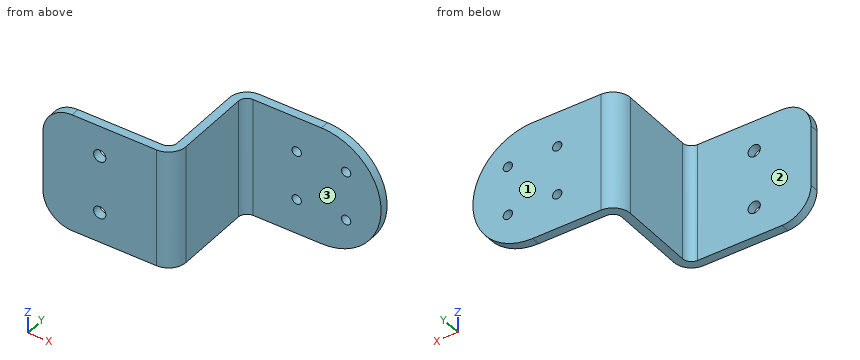
from build123d import *

# Parameters (mm, degrees)
EXTRUDE_THIN1_DEPTH    = 41
CONVERT_SOLID1_DEPTH   = 41
CONVERT_SOLID1_2_DEPTH = 41
SKETCH6_R              = 1.6
CUT_EXTRUDE1_DEPTH     = 3
M5X0_8_TAPPED_HOLE1_D  = 4.2
FILLET1_R              = 10


# Read off the part's stored shape, not the designer's step: Convert-Solid1
with BuildPart() as part:
    # Sketch1 → Extrude-Thin1 (new body)
    with BuildSketch(Plane.XY):
        Polygon((50, 35), (0, 35), (0, 0), (-45, 0), (-45, 3), (-3, 3), (-3, 38), (50, 38), align=None)
    extrude(amount=EXTRUDE_THIN1_DEPTH)

    # Convert-Solid1 outline → Convert-Solid1 (cut)
    with BuildSketch(Plane.XY):
        with BuildLine():
            Line((-3, 38), (-3, 32))
            ThreePointArc((-3, 32), (-1.242640687, 36.242640687), (3, 38))
            Line((3, 38), (-3, 38))
        make_face()
        with BuildLine():
            Line((0, 0), (0, 6))
            ThreePointArc((0, 6), (-1.757359313, 1.757359313), (-6, 0))
            Line((-6, 0), (0, 0))
        make_face()
    extrude(amount=CONVERT_SOLID1_DEPTH, mode=Mode.SUBTRACT)

    # Convert-Solid1 2 outline → Convert-Solid1 2 (add)
    with BuildSketch(Plane.XY):
        with BuildLine():
            Line((-3, 3), (-3, 6))
            ThreePointArc((-3, 6), (-3.878679656, 3.878679656), (-6, 3))
            Line((-6, 3), (-3, 3))
        make_face()
        with BuildLine():
            Line((0, 35), (0, 32))
            ThreePointArc((0, 32), (0.878679656, 34.121320344), (3, 35))
            Line((3, 35), (0, 35))
        make_face()
    extrude(amount=CONVERT_SOLID1_2_DEPTH)

    # Sketch6 → Cut-Extrude1 (cut)
    with BuildSketch(Plane(origin=(0, 38, 0), x_dir=(1, 0, 0), z_dir=(0, 1, 0))):
        with Locations(Location((34.985281374, -12.014718626, 0), (0, 0, 270))):
            Circle(SKETCH6_R)
        with Locations(Location((34.985281374, -28.985281374, 0), (0, 0, 270))):
            Circle(SKETCH6_R)
        with Locations(Location((18.014718626, -28.985281374, 0), (0, 0, 270))):
            Circle(SKETCH6_R)
        with Locations(Location((18.014718626, -12.014718626, 0), (0, 0, 270))):
            Circle(SKETCH6_R)
        with BuildLine():
            Line((51.105144577, 0), (51.105144577, -41))
            Line((51.105144577, -41), (26.5, -41))
            ThreePointArc((26.5, -41), (47, -20.5), (26.5, 0))
            Line((26.5, 0), (51.105144577, 0))
        make_face()
    extrude(amount=-CUT_EXTRUDE1_DEPTH, mode=Mode.SUBTRACT)

    # M5x0.8 Tapped Hole1 (through all)
    with Locations(Plane(origin=(0, 3, 0), x_dir=(1, 0, 0), z_dir=(0, 1, 0))):
        with Locations((-25.5, -30.5), (-25.5, -10.5)):
            Hole(M5X0_8_TAPPED_HOLE1_D / 2)

    # Fillet1
    fillet1_edges = [part.edges().sort_by_distance(p)[0] for p in [
        (-45, 1.5, 41),
        (-45, 1.5, 0),
    ]]
    fillet(fillet1_edges, radius=FILLET1_R)


solid = part.part
Design review of the part built by this model. Coordinates are the model's own, in mm. Face numbers are marked on the shaded views. A direction names the side the tool comes from. Give positions to 0.01 mm unless a question says otherwise; leave off trailing zeros. Loops run counter-clockwise (first coordinate to the right, second up) from the corner with the lowest first, then second, coordinate; pieces in that order, holes last. Notation, with made-up numbers: (66, 50) - (106, 50) arc R21 cw to (106, 87) - close; hole circle Ø10 at (74.25, 78.5). An arc over 180 degrees is marked (long way). Use CSV: the item, a comma, the result in double quotes. Start each with the question number.
1. Machinability: for the marked faces 1, 2 and 3, which of the approach directions +Z, -Z, +X, -X, +Y, -Y give a long, thin tool a straight path to every point of the face, cutting with its end or side? Answer none if there is none.
2. Add section C-C (y = 8). State the section outline as (x, z) points.
3. Wall thickness on L1, parallel to Z at x = -25.5, y = 2.3; L2, parallel to Z at x = -25, y = 2; L3, parallel to Y at x = -40, z = 37: over which ranges is each line inside the solid? List them lowest first.
4. Add section A-A (x = -25.5). State the section outline as (y, z) points.
5. Insertion check: P1, Ø8, axis at x = -16, z = 10.5, coming from the +Y side; P2, Ø13, axis at y = 20.5, z = 22.5, coming from the +X side; P3, Ø10, axis at y = 33, z = 23.5, coming from the -X side. Each pin has a flat end and moves straight along its axis. Give the tip position at first contact, or say it passes through.
6. Add section D-D (x = 25.5). State the section outline as (y, z) points.
7. Add section B-B (z = 20.5). State the section outline as (x, y) points, plus the area to 3 significant figures.
Results found:
1,face 1,"+Z, -Z, +X, -X, +Y"
1,face 2,"+Z, -Z, -X, +Y"
1,face 3,"+Z, -Z, +X, -Y"
2,outline,"(-3, 0) - (0, 0) - (0, 41) - (-3, 41) - close"
3,L1,"z = 0 to 8.4, 12.6 to 28.4, 32.6 to 41"
3,L2,"z = 0 to 8.46, 12.54 to 28.46, 32.54 to 41"
3,L3,"y = 0 to 3"
4,outline,"(0, 0) - (3, 0) - (3, 8.4) - (0, 8.4) - close; (0, 12.6) - (3, 12.6) - (3, 28.4) - (0, 28.4) - close; (0, 32.6) - (3, 32.6) - (3, 41) - (0, 41) - close"
5,P1,"stops at y = 3"
5,P2,"stops at x = 0"
5,P3,"stops at x = -3"
6,outline,"(35, 0) - (38, 0) - (38, 41) - (35, 41) - close"
7,outline,"(-45, 0) - (-6, 0) arc R6 ccw to (0, 6) - (0, 32) arc R3 cw to (3, 35) - (47, 35) - (47, 38) - (3, 38) arc R6 ccw to (-3, 32) - (-3, 6) arc R3 cw to (-6, 3) - (-45, 3) - close"
7,area,"369 mm²"
